Read the model definition and answer for the solid it produces. Units are mm, in the model's axes. A direction names the side the tool comes from. Give positions to 0.01 mm unless a question says otherwise; leave off trailing zeros. Loops run counter-clockwise (first coordinate to the right, second up) from the corner with the lowest first, then second, coordinate; pieces in that order, holes last. Notation, with made-up numbers: M 14.5,78 L 19.5,78 A19 cw 19.5,97 Z; hole C 20,54.5 d2. An arc over 180 degrees is marked long. Return JSON: item names as keys, results as strings. Group by question number.
Autodesk Inventor part; units mm, degrees
ref_plane "YZ Plane" through (0, 0, 0) normal (1, 0, 0) x (0, 1, 0)
ref_plane "XZ Plane" through (0, 0, 0) normal (0, 1, 0) x (-1, 0, 0)
ref_plane "XY Plane" through (0, 0, 0) normal (0, 0, 1) x (1, 0, 0)
sketch "Sketch1" plane through (0, 0, 0) normal (0, 0, 1) x (1, 0, 0)
  line L0 (10.8783, -7.0389) -> (-10.8783, -7.0389)
  line L1 (-10.8783, -7.0389) -> (-10.8783, 7.0389)
  line L2 (-10.8783, 7.0389) -> (10.8783, 7.0389)
  line L3 (10.8783, 7.0389) -> (10.8783, -7.0389)
  line L4 (10.8783, -7.0389) -> (-10.8783, 7.0389) construction
  line L5 (-10.8783, -7.0389) -> (10.8783, 7.0389) construction
  point P0 (0, 0)
extrude "Extrusion1" add sketch "Sketch1" along normal blind 9
sketch "Sketch2" plane through (-10.8783, 7.0389, 0) normal (0, 1, 0) x (1, 0, 0)
  circle A0 centre (4.2234, -4.5433) radius 1.9026
  circle A1 centre (18.0126, -4.5433) radius 1.9371
  point P0 (10.8783, 0)
extrude "Extrusion2" cut sketch "Sketch2" against normal blind 2
sketch "Sketch3" plane through (10.8783, -7.0389, 0) normal (1, 0, 0) x (0, 0, -1)
  circle A0 centre (-4.4153, 7.0389) radius 1.5998
  point P0 (0, 7.0389)
extrude "Extrusion3" cut sketch "Sketch3" against normal blind 2
sketch "Sketch4" plane through (-10.8783, -7.0389, 0) normal (0, -1, 0) x (1, 0, 0)
  circle A0 centre (18.0126, 4.5433) radius 1.9371
  circle A1 centre (18.0126, 4.5433) radius 1.9371
  circle A2 centre (3.4358, 4.4153) radius 2.0338
  point P0 (10.8783, 0)
extrude "Extrusion4" cut sketch "Sketch4" against normal blind 2
properties part number "body_of_the_bot"
1. Find section B-B (z = 5.5). Write down the section's boundary in (x, y).
2. Find section A-A (y = 1). Write down the section's boundary in (x, z).
3. Flat-ended cylindrical pins translate along their axes: P1, Ø2.5, axis at y = 0, z = 5, coming from the +X side; P2, Ø3.5, axis at x = 7.13, z = 4.54, coming from the -Y side; P3, Ø1.9, axis at x = -6.5, z = 4.5, coming from the +Y side. Find the tip coordinate at first contact, or state that the pin passes through.
4. For faces 1 (the cylindrical face through (5.707, -6.053, 5.852)), 2 (the cylindrical face through (9.892, -0.613, 2.937)), 3 (the flat face through (7, 5.039, 5)), determine the directions among +Z, -Z, +X, -X, +Y, -Y from which every point of the face is accessible in a straight line to the end or side of a thin tool.
5. Find section C-C (z = 3.75). Write down the section's boundary in (x, y).
6. Straight lines are drawn through the part: line 1 along X through (y, z) = (5.75, 3.5); line 2 along X through (y, z) = (-5.25, 3.75); line 3 along X through (y, z) = (-0.5, 4). For each, find the intervals that lie inside material, in ascending order.
7. The mould has two halves that part along Z. Classify faces 4 (the flat face through (0, 0, 0)), 5 (the flat face through (0, -7.039, 4)), 6 (the cylindrical face through (-5.564, -6.053, 3.636)): +Z half, -Z half, draft (parallel to the pull), parting line (faces both ways), or undercut.
Result:
{
 "1": {"outline": "M -10.88,-7.04 L -9.16,-7.04 L -9.16,-5.04 L -5.72,-5.04 L -5.72,-7.04 L 5.45,-7.04 L 5.45,-5.04 L 8.82,-5.04 L 8.82,-7.04 L 10.88,-7.04 L 10.88,-1.18 L 8.88,-1.18 L 8.88,1.18 L 10.88,1.18 L 10.88,7.04 L 8.82,7.04 L 8.82,5.04 L 5.45,5.04 L 5.45,7.04 L -5.01,7.04 L -5.01,5.04 L -8.3,5.04 L -8.3,7.04 L -10.88,7.04 Z"},
 "2": {"outline": "M -10.88,0 L 10.88,0 L 10.88,3.17 L 8.88,3.17 L 8.88,5.66 L 10.88,5.66 L 10.88,9 L -10.88,9 Z"},
 "3": {"P1": "stops at x = 10.88", "P2": "stops at y = -5.04", "P3": "stops at y = 5.04"},
 "4": {"face 1": "-Y", "face 2": "+X", "face 3": "+Y"},
 "5": {"outline": "M -10.88,-7.04 L -9.36,-7.04 L -9.36,-5.04 L -5.52,-5.04 L -5.52,-7.04 L 5.37,-7.04 L 5.37,-5.04 L 8.9,-5.04 L 8.9,-7.04 L 10.88,-7.04 L 10.88,-1.45 L 8.88,-1.45 L 8.88,1.45 L 10.88,1.45 L 10.88,7.04 L 8.9,7.04 L 8.9,5.04 L 5.37,5.04 L 5.37,7.04 L -4.93,7.04 L -4.93,5.04 L -8.38,5.04 L -8.38,7.04 L -10.88,7.04 Z"},
 "6": {"line 1": "x = -10.88 to -8.25, -5.06 to 5.5, 8.77 to 10.88", "line 2": "x = -10.88 to -9.36, -5.52 to 5.37, 8.9 to 10.88", "line 3": "x = -10.88 to 8.88"},
 "7": {"face 4": "-Z half", "face 5": "draft", "face 6": "undercut"}
}
